Solid Edge part; units mm, degrees
sketch "Sketch1" plane through (0, 0, 0) normal (0, -1, 0) x (1, 0, 0)
  circle A0 centre (0, 0) radius 16.5
extrude "Protrusion1" add sketch "Sketch1" against normal blind 1.5
sketch "Sketch2" plane through (0, 0, 0) normal (0, -1, 0) x (1, 0, 0)
  circle A0 centre (0, 0) radius 15
extrude "ProtrusiónExtruida_2" add sketch "Sketch2" along normal blind 17.5
sketch "Sketch3" plane through (0, -17.5, 0) normal (0, -1, 0) x (1, 0, 0)
  circle A0 centre (0, 0) radius 7.5
extrude "ProtrusiónExtruida_3" add sketch "Sketch3" along normal blind 6
sketch "Sketch4" plane through (0, -23.5, 0) normal (0, -1, 0) x (1, 0, 0)
  line L0 (5, -5) -> (-5, -5)
  line L1 (-5, -5) -> (-5, 5)
  line L2 (-5, 5) -> (5, 5)
  line L3 (5, 5) -> (5, -5)
  dimension "D1" = 5
  dimension "D2" = 5
extrude "ProtrusiónExtruida_4" add sketch "Sketch4" along normal blind 14
sketch "Sketch5" plane through (0, 1.5, 0) normal (0, 1, 0) x (0, 0, -1)
  circle A0 centre (0, 0) radius 16.5
extrude "ProtrusiónExtruida_5" add sketch "Sketch5" along normal blind 0.54
hole "Agujero_1" at (-11, -17.5, 0) direction (0, 1, 0) diameter 3 end up to next counterbore diameter 5 counterbore depth 16
pattern_circular "Pattern1" count 8 over 360 about axis through (0, -17.5, 0) along (0, 1, 0) of "Agujero_1"
sketch "Sketch6" plane through (0, 1.5, 0) normal (0, 1, 0) x (0, 0, -1)
  circle A0 centre (0, 0) radius 5
extrude "VaciadoExtruido_1" cut sketch "Sketch6" along normal mid plane 12
fillet "Redondeo_1" radius 1 4 edges at (-5, -30.5, -5) (-5, -30.5, 5) (5, -30.5, 5) (5, -30.5, -5)
hole "Agujero_9" at (0, -37.5, 0) direction (0, 1, 0) diameter 4.917 depth 20 tip angle 118 thread major 6 thread length 18
sketch "Sketch7" plane through (0, 2.04, 0) normal (0, 1, 0) x (0, 0, 1)
  circle A0 centre (0, 0) radius 16.5
extrude "VaciadoExtruido_2" cut sketch "Sketch7" against normal blind 0.04
properties part number "1976-1200-012" material "Aluminio, 7075-T6"
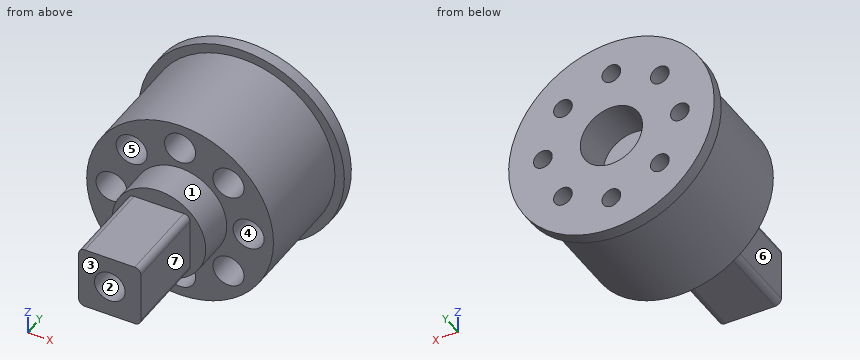
Verification items for the finished model (mm, model axes). Face numbers are marked on the shaded views. A direction names the side the tool comes from. Give positions to 0.01 mm unless a question says otherwise; leave off trailing zeros. Write each loop counter-clockwise with the first axis right and the second up, starting at its lowest first coordinate (ties: lowest second). Pieces come first, ordered by that corner, then holes. Notation, with made-up numbers: (74.25, -14.75) - (86.25, -14.75) arc R16 ccw to (86.25, -5.75) - close; hole circle Ø3 at (35.25, 48). An arc over 180 degrees is marked (long way). Put each result on its own line as item: value.
Q1. Depth check by flat-ended pin: P1, Ø6.5, axis at x = 1.5, y = -33.5, coming from the +Z side; P2, Ø1.5, axis at x = 8.5, z = 6.5, coming from the -Y side; P3, Ø6, axis at x = -8, y = -19, coming from the +Z side; P4, Ø10, axis at y = -23.5, z = -13, coming from the +X side. Enter the tip coordinate at first touch or a pass-through.
Result:
P1: z = 5
P2: y = -1.5
P3: z = 13.99
P4: through
Q2. Section check C-C on y = -5. Count the separate pieces of the cut face and the enclosed holes in it, and give its area (3 significant figures).
Result:
separate pieces: 1
enclosed holes: 8
area: 550 mm2
Q3. Set-up check for the marked faces 5, 6 and 7: record each of +Z, -Z, +X, -X, +Y, -Y from which the full face is reachable in a straight line by a thin tool's end or side.
Result:
face 5: -Y
face 6: +Z, -Z, -X, -Y
face 7: +Z, -Z, +X, -Y
Q4. Section check D-D on x = -3. Record the cut outline in (y, z).
Result:
outline: (-37.5, -5) - (-23.5, -5) - (-23.5, -6.87) - (-17.5, -6.87) - (-17.5, -14.7) - (0, -14.7) - (0, -16.22) - (2, -16.22) - (2, -4) - (-4.5, -4) - (-4.5, 4) - (2, 4) - (2, 16.22) - (0, 16.22) - (0, 14.7) - (-17.5, 14.7) - (-17.5, 6.87) - (-23.5, 6.87) - (-23.5, 5) - (-37.5, 5) - close
Q5. Mould release check, pull along X, two halves, no side actions. Record for the marked faces 1, 2, 3 and 4: released by +X, released by -X, zero draft, split by the parting line, or undercut.
Result:
face 1: split by the parting line
face 2: undercut
face 3: zero draft
face 4: undercut
Q6. Section check B-B on y = -29.5. Record the cut outline in (x, z), and give its area (3 significant figures).
Result:
outline: (-5, -4) arc R1 ccw to (-4, -5) - (4, -5) arc R1 ccw to (5, -4) - (5, 4) arc R1 ccw to (4, 5) - (-4, 5) arc R1 ccw to (-5, 4) - close; hole circle Ø4.92 at (0, 0)
area: 80.2 mm2
Q7. Section check A-A on x = -11. Record the cut outline in (y, z).
Result:
outline: (-17.5, -10.2) - (0, -10.2) - (0, -12.3) - (2, -12.3) - (2, -1.5) - (-1.5, -1.5) - (-1.5, -2.5) - (-17.5, -2.5) - close; (-17.5, 2.5) - (-1.5, 2.5) - (-1.5, 1.5) - (2, 1.5) - (2, 12.3) - (0, 12.3) - (0, 10.2) - (-17.5, 10.2) - close
Q8. Scan lines: probe 1 along Z at (x, y) = (0, -6); probe 2 along Z at (x, y) = (-5.5, -9.5); probe 3 along Z at (x, y) = (0, -27). Record each from-to range of solid material in increasing order. Write a range as from..to.
Result:
probe 1: -15..-13.5, -8.5..8.5, 13.5..15
probe 2: -13.96..-8.81, -6.75..6.75, 8.81..13.96
probe 3: -5..-2.46, 2.46..5
